Read the model definition and answer for the solid it produces. Units are mm, in the model's axes. A direction names the side the tool comes from. Coordinates: 2 decimals unless noted, no trailing zeros. Order: outer loops, then holes, each group sorted by start corner. A loop starts at its lowest first (then second) coordinate and runs counter-clockwise, first axis right, second up.
```python
from build123d import *

# Parameters (mm, degrees)
SKETCH_1_W          = 49
SKETCH_1_H          = 40
EXTRUDE_1_DEPTH     = 4
SKETCH_2_R          = 1.5
CUT_EXTRUDE_1_DEPTH = 32.878676259
SKETCH_3_W          = 10
SKETCH_3_H          = 30
EXTRUDE_3_DEPTH     = 40
SKETCH_4_R          = 5.2
CUT_EXTRUDE_2_DEPTH = 69.82586723
SKETCH_5_R          = 11.75
CUT_EXTRUDE_3_DEPTH = 5
SKETCH_6_R          = 1.5
CUT_EXTRUDE_4_DEPTH = 66.360538553
EXTRUDE_4_DEPTH     = 6
SKETCH_8_W          = 6
SKETCH_8_H          = 64
EXTRUDE_5_DEPTH     = 49
SKETCH_9_R          = 1.6
CUT_EXTRUDE_5_DEPTH = 80.348913036
EXTRUDE_6_DEPTH     = 5
SKETCH_12_W         = 49
SKETCH_12_H         = 6
EXTRUDE_7_DEPTH     = 90
SKETCH_13_R         = 1.6
CUT_EXTRUDE_6_DEPTH = 161.985247771
EXTRUDE_8_DEPTH     = 5


with BuildPart() as part:
    # 草图1 → 凸台-拉伸1 (new body)
    with BuildSketch(Plane(origin=(0, 0, 0), x_dir=(1, 0, 0), z_dir=(0, 1, 0))):
        Rectangle(SKETCH_1_W, SKETCH_1_H)
    extrude(amount=EXTRUDE_1_DEPTH)

    # 草图2 → 切除-拉伸1 (cut, through all)
    with BuildSketch(Plane(origin=(0, 4, 0), x_dir=(1, 0, 0), z_dir=(0, 1, 0))):
        with Locations(Location((-10, 10, 0), (0, 0, 270))):
            Circle(SKETCH_2_R)
        with Locations(Location((10, 10, 0), (0, 0, 270))):
            Circle(SKETCH_2_R)
        with Locations(Location((10, -10, 0), (0, 0, 270))):
            Circle(SKETCH_2_R)
        with Locations(Location((-10, -10, 0), (0, 0, 270))):
            Circle(SKETCH_2_R)
    extrude(amount=-CUT_EXTRUDE_1_DEPTH, mode=Mode.SUBTRACT)

    # 草图3 → 凸台-拉伸3 (add)
    with BuildSketch(Plane(origin=(0, 4, 0), x_dir=(1, 0, 0), z_dir=(0, 1, 0))):
        with Locations((-19.5, 0)):
            Rectangle(SKETCH_3_W, SKETCH_3_H)
    extrude(amount=EXTRUDE_3_DEPTH)

    # 草图4 → 切除-拉伸2 (cut, through all)
    with BuildSketch(Plane.ZY.offset(24.5)):
        with Locations((0, 28)):
            Circle(SKETCH_4_R)
    extrude(amount=-CUT_EXTRUDE_2_DEPTH, mode=Mode.SUBTRACT)

    # 草图5 → 切除-拉伸3 (cut)
    with BuildSketch(Plane.ZY.offset(24.5)):
        with Locations((0, 28)):
            Circle(SKETCH_5_R)
    extrude(amount=-CUT_EXTRUDE_3_DEPTH, mode=Mode.SUBTRACT)

    # 草图6 → 切除-拉伸4 (cut, through all)
    with BuildSketch(Plane.ZY.offset(19.5)):
        with Locations((-5.656854249, 33.656854249)):
            Circle(SKETCH_6_R)
        with Locations((5.656854249, 33.656854249)):
            Circle(SKETCH_6_R)
        with Locations((5.656854249, 22.343145751)):
            Circle(SKETCH_6_R)
        with Locations((-5.656854249, 22.343145751)):
            Circle(SKETCH_6_R)
    extrude(amount=-CUT_EXTRUDE_4_DEPTH, mode=Mode.SUBTRACT)

    # 草图7 → 凸台-拉伸4 (add, symmetric)
    with BuildSketch(Plane(origin=(0, 0, 0), x_dir=(-1, 0, 0), z_dir=(0, 0, -1))):
        Polygon((14.5, 17), (-24.5, 4), (14.5, 4), align=None)
    extrude(amount=EXTRUDE_4_DEPTH, both=True)

    # 草图8 → 凸台-拉伸5 (add)
    with BuildSketch(Plane.ZY.offset(24.5)):
        with Locations((17, -32)):
            Rectangle(SKETCH_8_W, SKETCH_8_H)
        with Locations((-17, -32)):
            Rectangle(SKETCH_8_W, SKETCH_8_H)
    extrude(amount=-EXTRUDE_5_DEPTH)

    # 草图9 → 切除-拉伸5 (cut, through all)
    with BuildSketch(Plane.XY.offset(20)):
        with Locations((20.5, -60)):
            Circle(SKETCH_9_R)
        with Locations((-20.5, -60)):
            Circle(SKETCH_9_R)
        with Locations((20.5, -38)):
            Circle(SKETCH_9_R)
        with Locations((-20.5, -38)):
            Circle(SKETCH_9_R)
    extrude(amount=-CUT_EXTRUDE_5_DEPTH, mode=Mode.SUBTRACT)

    # 草图11 → 凸台-拉伸6 (add)
    with BuildSketch(Plane.XY.offset(15)):
        Polygon((-14.5, 44), (24.5, 9), (24.5, 4), (-14.5, 4), (-24.5, 4), (-24.5, 44), align=None)
    extrude_6 = extrude(amount=EXTRUDE_6_DEPTH)

    # 镜向2: 凸台-拉伸6 across plane
    add(extrude_6.mirror(Plane(origin=(0, 0, 0), x_dir=(1, 0, 0), z_dir=(0, 0, -1))))

    # 草图12 → 凸台-拉伸7 (add)
    with BuildSketch(Plane.XZ.offset(64)):
        with Locations((0, -17)):
            Rectangle(SKETCH_12_W, SKETCH_12_H)
    extrude(amount=EXTRUDE_7_DEPTH)

    # 草图13 → 切除-拉伸6 (cut, through all)
    with BuildSketch(Plane(origin=(0, 0, -20), x_dir=(-1, 0, 0), z_dir=(0, 0, -1))):
        with Locations((-20.5, -120)):
            Circle(SKETCH_13_R)
        with Locations((-20.5, -142)):
            Circle(SKETCH_13_R)
        with Locations((20.5, -120)):
            Circle(SKETCH_13_R)
        with Locations((20.5, -142)):
            Circle(SKETCH_13_R)
    extrude(amount=-CUT_EXTRUDE_6_DEPTH, mode=Mode.SUBTRACT)

    # 草图14 → 凸台-拉伸8 (add, symmetric)
    with BuildSketch(Plane(origin=(0, 0, 0), x_dir=(0, 0, -1), z_dir=(1, 0, 0))):
        Polygon((14, 0), (-14, 0), (-14, -64), (9, -154), (14, -154), (14, -64), align=None)
    extrude(amount=EXTRUDE_8_DEPTH, both=True)


solid = part.part
```
1) Straight lines are drawn through the part: line 1 (Z direction, x = -15, y = 22); line 2 (X direction, y = -142, z = -18.6); line 3 (Z direction, x = -1, y = 10). For each, find the intervals that lie inside material, in ascending order.
A:
line 1: z = -20 to -7.12, -4.2 to 4.2, 7.12 to 20
line 2: x = -24.5 to -22.1, -18.9 to 18.9, 22.1 to 24.5
line 3: z = -20 to -15, -6 to 6, 15 to 20
2) Flat-ended cylindrical pins translate along their axes: pin 1 Ø1.5 at (y, z) = (-17, 11) entering from +X; pin 2 Ø6.5 at (x, z) = (8.5, 16) entering from -Y; pin 3 Ø10 at (x, z) = (2.5, 12.5) entering from +Y. Find the tip coordinate at first contact, or state that the pin passes through.
A:
pin 1: stops at x = 5
pin 2: stops at y = -64
pin 3: stops at y = 32.63
3) A cutting plane is placed at C-C, the plane x = 17. Determine the outline of the cut face in (y, z).
A:
outline: (-154, -20) - (15.73, -20) - (15.73, -15) - (4, -15) - (4, -6) - (6.5, -6) - (6.5, 6) - (4, 6) - (4, 15) - (15.73, 15) - (15.73, 20) - (-64, 20) - (-64, 14) - (0, 14) - (0, -14) - (-154, -14) - close
4) A cutting plane is placed at B-B, the plane y = -4. Determine the outline of the cut face in (x, z), and give its area (3 significant figures).
A:
outline: (-24.5, -20) - (24.5, -20) - (24.5, -14) - (5, -14) - (5, 14) - (24.5, 14) - (24.5, 20) - (-24.5, 20) - (-24.5, 14) - (-5, 14) - (-5, -14) - (-24.5, -14) - close
area: 868 mm2
5) A cutting plane is placed at D-D, the plane y = -133.5. Determine the outline of the cut face in (x, z), and give its area (3 significant figures).
A:
outline: (-24.5, -20) - (24.5, -20) - (24.5, -14) - (5, -14) - (5, -3.76) - (-5, -3.76) - (-5, -14) - (-24.5, -14) - close
area: 396 mm2
6) Determine the mould class of faces 4 (the flat face through (-20, 44, 0)), 5 (the flat face through (1, 20, -15)), 6 (the flat face through (0.07, -108.37, 2.66)), 7 (the cylindrical face through (-17.035, 22.924, -1.127)) for opening direction Z: pulls with the +Z half, pulls with the -Z half, needs draft (parallel to the pull), parting line crosses it, or undercut.
A:
face 4: needs draft
face 5: undercut
face 6: pulls with the +Z half
face 7: undercut
7) A cutting plane is placed at A-A, the plane z = 0. Determine the outline of the cut face in (x, y).
A:
outline: (-24.5, 0) - (-5, 0) - (-5, -118.78) - (5, -118.78) - (5, 0) - (24.5, 0) - (24.5, 4) - (-14.5, 17) - (-14.5, 22.8) - (-19.5, 22.8) - (-19.5, 16.25) - (-24.5, 16.25) - close; (-24.5, 39.75) - (-19.5, 39.75) - (-19.5, 33.2) - (-14.5, 33.2) - (-14.5, 44) - (-24.5, 44) - close
8) Which of the six approach directions +Z, -Z, +X, -X, +Y, -Y give full straight-line access (tool end or side, diameter ignored) to faces 1 (the flat face through (-24.5, -25, -15)), 2 (the flat face through (-3, 8, 6)), 3 (the cylindrical face through (-22.04, 39.65, -1.53))?
A:
face 1: +Z, -Z, -X, +Y, -Y
face 2: +X, +Y
face 3: -X
